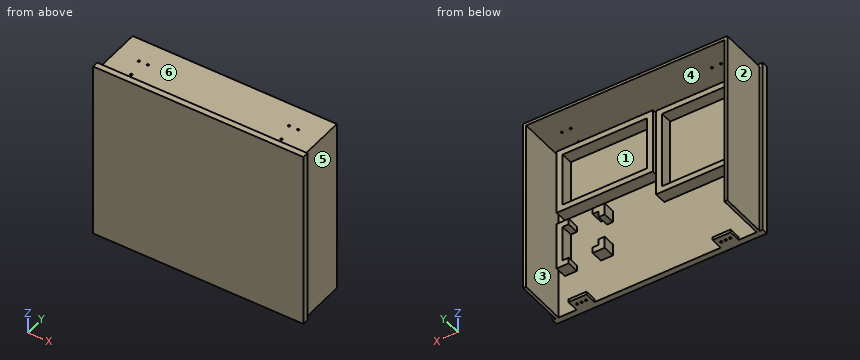
Autodesk Inventor part; units mm, degrees
ref_plane "YZ Plane" through (0, 0, 0) normal (1, 0, 0) x (0, 1, 0)
ref_plane "XZ Plane" through (0, 0, 0) normal (0, 1, 0) x (-1, 0, 0)
ref_plane "XY Plane" through (0, 0, 0) normal (0, 0, 1) x (1, 0, 0)
sketch "Sketch1" plane through (0, 0, 0) normal (0, 1, 0) x (-1, 0, 0)
  line L0 (-175, 150) -> (175, 150)
  line L1 (175, 150) -> (175, -150)
  line L2 (175, -150) -> (-175, -150)
  line L3 (-175, -150) -> (-175, 150)
  line L4 (-175, 150) -> (175, -150) construction
  line L5 (175, 150) -> (-175, -150) construction
  point P0 (0, 0)
  dimension "d0" = 350
  dimension "d1" = 300
extrude "Extrusion1" add sketch "Sketch1" along normal blind 10
sketch "Sketch2" plane through (0, 10, 0) normal (0, 1, 0) x (1, 0, 0)
  line L0 (175, 150) -> (-175, 150)
  line L1 (-175, 150) -> (-170, 150)
  line L2 (-170, 150) -> (-165, 150)
  line L3 (-165, 150) -> (-165, -145)
  line L4 (-165, -145) -> (-170, -145)
  line L5 (-170, -145) -> (-170, 150)
  line L6 (-170, -145) -> (170, -145)
  line L7 (170, -145) -> (170, -140)
  line L8 (170, -140) -> (-170, -140)
  line L9 (-170, -140) -> (-170, -145)
  line L10 (170, -140) -> (165, -140)
  line L11 (165, -140) -> (165, 150)
  line L12 (165, 150) -> (170, 150)
  line L13 (170, 150) -> (170, -140)
  point P0 (0, 0)
  point P1 (-170, 145)
  point P2 (170, 145)
  point P3 (-165, -140)
  point P4 (-165, -145)
  dimension "d5" = 5
  dimension "d6" = 5
  dimension "d7" = 5
extrude "Extrusion2" add sketch "Sketch2" along normal blind 80 contours L13 L8 L11 L0 | L7 L6 L3 L8 | L3 L8 L5 L0 | L3 L4 L5 L8
sketch "Sketch3" plane through (-175, 0, 150) normal (0, 0, 1) x (1, 0, 0)
  line L0 (5, 10) -> (5, 90)
  line L1 (5, 90) -> (50, 90)
  line L2 (340, 90) -> (10, 90)
  line L3 (50, 90) -> (50, 20)
  line L4 (345, 10) -> (345, 90)
  line L5 (345, 90) -> (300, 90)
  line L6 (300, 90) -> (300, 20)
  line L7 (350, 10) -> (345, 10)
  line L8 (350, 10) -> (350, 90)
  point P0 (175, 0)
  point P1 (307.5, 50)
  point P2 (292.5, 50)
  point P3 (42.5, 50)
  point P4 (57.5, 50)
  dimension "d10" = 45
  dimension "d11" = 70
  dimension "d12" = 45
  dimension "d13" = 70
sketch "Sketch4" plane through (0, 10, 0) normal (0, 1, 0) x (1, 0, 0)
  line L0 (165, 150) -> (-165, 150)
  line L1 (-165, 150) -> (-135, 150)
  line L2 (-135, 150) -> (-105, 150)
  line L3 (-105, 150) -> (-105, 145)
  line L4 (-105, 145) -> (-135, 145)
  line L5 (-135, 145) -> (-135, 150)
  line L6 (165, 150) -> (135, 150)
  line L7 (135, 150) -> (105, 150)
  line L8 (105, 150) -> (105, 145)
  line L9 (105, 145) -> (135, 145)
  line L10 (135, 145) -> (135, 150)
  point P0 (0, 0)
  dimension "d21" = 30
  dimension "d22" = 30
  dimension "d23" = 5
  dimension "d24" = 30
  dimension "d25" = 30
  dimension "d26" = 5
extrude "Extrusion3" add sketch "Sketch4" along normal blind 20
sketch "Sketch5" plane through (175, 0, -150) normal (0, 0, -1) x (-1, 0, 0)
  circle A0 centre (295, 20) radius 1.75
  line L0 (287.5, 20) -> (295, 20)
  point P0 (175, 0)
  point P1 (302.5, 20)
  point P2 (55, 20)
  point P3 (62.5, 20)
  point P4 (47.5, 20)
  dimension "d45" = 7.5
hole "Hole2" at (-120, 20, -150) at (-127.5, 20, -150) at (-112.5, 20, -150) at (120, 20, -150) at (112.5, 20, -150) at (127.5, 20, -150) direction (0, 0, 1) diameter 3.5 depth 10
hole "Hole3" at (-125, 20, 150) at (125, 20, 150) at (132.5, 50, 150) at (117.5, 50, 150) at (-132.5, 50, 150) at (-117.5, 50, 150) direction (0, 0, -1) diameter 3.5 depth 10
sketch "Sketch6" plane through (0, 10, 0) normal (0, 1, 0) x (1, 0, 0)
  line L0 (-165, -140) -> (165, -140)
  line L1 (165, -140) -> (215, -140) construction
  line L2 (-5.3553, -129.6447) -> (154.6447, -129.6447)
  line L3 (154.6447, -129.6447) -> (154.6447, -19.6447)
  line L4 (154.6447, -19.6447) -> (-5.3553, -19.6447)
  line L5 (-5.3553, -19.6447) -> (-5.3553, -129.6447)
  line L6 (-5.3553, -129.6447) -> (154.6447, -19.6447) construction
  line L7 (154.6447, -129.6447) -> (-5.3553, -19.6447) construction
  line L8 (4.6447, -119.6447) -> (144.6447, -119.6447)
  line L9 (144.6447, -119.6447) -> (144.6447, -29.6447)
  line L10 (144.6447, -29.6447) -> (4.6447, -29.6447)
  line L11 (4.6447, -29.6447) -> (4.6447, -119.6447)
  line L12 (4.6447, -119.6447) -> (144.6447, -29.6447) construction
  line L13 (144.6447, -119.6447) -> (4.6447, -29.6447) construction
  point P0 (0, 0)
  point P1 (74.6447, -74.6447)
  dimension "d51" = 160
  dimension "d52" = 110
  dimension "d70" = 140
  dimension "d71" = 90
sketch "Sketch7" plane through (0, 10, 0) normal (0, 1, 0) x (1, 0, 0)
  line L0 (-165, -140) -> (165, -140)
  line L1 (-165, -140) -> (-150.8579, -125.8579)
  line L2 (-165, -140) -> (-145, -140) construction
  line L3 (-150.8579, -125.8579) -> (-10.8579, -125.8579)
  line L4 (-10.8579, -125.8579) -> (-10.8579, 24.1421)
  line L5 (-10.8579, 24.1421) -> (-150.8579, 24.1421)
  line L6 (-150.8579, 24.1421) -> (-150.8579, -125.8579)
  line L7 (-150.8579, -50.8579) -> (-80.8579, -50.8579)
  line L8 (-140.8579, -115.8579) -> (-20.8579, -115.8579)
  line L9 (-20.8579, -115.8579) -> (-20.8579, 14.1421)
  line L10 (-20.8579, 14.1421) -> (-140.8579, 14.1421)
  line L11 (-140.8579, 14.1421) -> (-140.8579, -115.8579)
  line L12 (-140.8579, -115.8579) -> (-20.8579, 14.1421) construction
  line L13 (-20.8579, -115.8579) -> (-140.8579, 14.1421) construction
  line L14 (-140.8579, -115.8579) -> (-150.8579, -115.8579)
  line L15 (-5.3553, -19.6447) -> (154.6447, -19.6447)
  line L16 (154.6447, -19.6447) -> (154.6447, 0.3553)
  line L17 (154.6447, 0.3553) -> (74.6447, 0.3553)
  line L18 (74.6447, 0.3553) -> (74.6447, 80.3553)
  line L19 (74.6447, 80.3553) -> (154.6447, 80.3553)
  line L20 (154.6447, 80.3553) -> (154.6447, 0.3553)
  line L21 (84.6447, 70.3553) -> (144.6447, 70.3553)
  line L22 (144.6447, 70.3553) -> (144.6447, 10.3553)
  line L23 (144.6447, 10.3553) -> (84.6447, 10.3553)
  line L24 (84.6447, 10.3553) -> (84.6447, 70.3553)
  line L25 (84.6447, 70.3553) -> (144.6447, 10.3553) construction
  line L26 (144.6447, 70.3553) -> (84.6447, 10.3553) construction
  line L27 (94.645, 70.3553) -> (134.645, 70.3553)
  line L28 (134.645, 70.3553) -> (134.645, 80.3553)
  line L29 (94.645, 80.3553) -> (94.645, 70.3553)
  line L30 (94.645, 10.3553) -> (134.645, 10.3553)
  line L31 (134.645, 0.3553) -> (94.645, 0.3553)
  line L32 (94.645, 80.3553) -> (134.645, 80.3553)
  line L33 (94.645, 10.3553) -> (94.645, 0.3553)
  line L34 (134.645, 10.3553) -> (94.645, 10.3553)
  line L35 (134.645, 10.3553) -> (134.645, 0.3553)
  line L36 (94.645, 0.3553) -> (134.645, 0.3553)
  line L37 (84.6447, 60.355) -> (84.6447, 20.355)
  line L38 (84.6447, 20.355) -> (74.6447, 20.355)
  line L39 (74.6447, 60.355) -> (84.6447, 60.355)
  point P0 (0, 0)
  point P1 (-140.8579, -50.8579)
  point P2 (114.6447, 40.3553)
  dimension "d55" = 20
  dimension "d56" = 45
  dimension "d57" = 140
  dimension "d58" = 150
  dimension "d59" = 120
  dimension "d60" = 130
  dimension "d61" = 20
  dimension "d62" = 80
  dimension "d63" = 80
  dimension "d75" = 60
  dimension "d76" = 60
  dimension "d77" = 40
  dimension "d78" = 40
extrude "Extrusion6" add sketch "Sketch6" along normal blind 20
extrude "Extrusion7" add sketch "Sketch7" along normal blind 20 contours L6 L14 L8 L9 L10 L11 L7 L5 L4 L3 | L17 L35 L23 L22 L21 L28 L19 L20 | L17 L18 L38 L24 L23 L33 | L29 L21 L24 L39 L18 L19
properties part number "Venstre_bottom"
Input: part model. Units: mm. Frame: model coordinates. Face numbers are marked on the shaded views. A direction names the side the tool comes from. Coordinates: 2 decimals unless noted, no trailing zeros. Write each loop counter-clockwise with the first axis right and the second up, starting at its lowest first coordinate (ties: lowest second). Pieces come first, ordered by that corner, then holes. Notation, with made-up numbers: M 75.25,58.5 L 124.25,58.5 A31 ccw 124.25,94.5 Z; hole C 4,41 d3. An arc over 180 degrees is marked long. Answer as a JSON object with one key per item and string values. Group by question number.
(1) Mould query, pull axis Z, two halves, no side actions, for the marked faces 4, 5 and 6. Classes: pulls with the +Z half, pulls with the -Z half, needs draft (parallel to the pull), parting line crosses it, or undercut.
(2) Section C-C on x = 17. Output: boundary loops of the cut face in (y, z), plus the area to 3 significant figures.
(3) Section D-D on z = -85. Output: boundary loops of the cut face in (x, y), plus the area to 3 significant figures.
(4) Ray query, line 1 along X through (y, z) = (27, 59); line 2 along Z through (x, y) = (31.5, 23); line 3 along X through (y, z) = (50, 141). Return the intervals inside material, ascending. Write a range as [from, to].
(5) Contact query for flat-ended pins moving along their axis: P1, Ø5.5, axis at x = 127.5, y = 20, coming from the +Z side; P2, Ø4.5, axis at x = -132.5, y = 50, coming from the -Z side; P3, Ø1.5, axis at x = -127, z = -147.5, coming from the +Y side. Output: stop coordinate, or through.
(6) Section A-A on z = 93. Output: boundary loops of the cut face in (x, y).
(7) Set-up query: the marked faces 1, 2 and 3. Return all of +Z, -Z, +X, -X, +Y, -Y with unobstructed straight access to the full face (end or side cutting, diameter ignored); none if empty.
(8) Section B-B on y = 42. Output: boundary loops of the cut face in (x, z).
Result set:
{
 "1": {"face 4": "undercut", "face 5": "needs draft", "face 6": "pulls with the +Z half"},
 "2": {"outline": "M 0,-150 L 10,-150 L 10,19.64 L 30,19.64 L 30,29.64 L 10,29.64 L 10,119.64 L 30,119.64 L 30,129.64 L 10,129.64 L 10,140 L 90,140 L 90,145 L 10,145 L 10,150 L 0,150 Z", "area": "3,800 mm2"},
 "3": {"outline": "M -175,0 L 175,0 L 175,10 L 170,10 L 170,90 L 165,90 L 165,10 L -165,10 L -165,90 L -170,90 L -170,10 L -175,10 Z", "area": "4,300 mm2"},
 "4": {"line 1": "x = [-170, -165], [-20.86, -10.86], [-5.36, 4.64], [144.64, 154.64], [165, 170]", "line 2": "z = [19.64, 29.64], [119.64, 129.64], [140, 145]", "line 3": "x = [-170, -134.25], [-130.75, -119.25], [-115.75, 115.75], [119.25, 130.75], [134.25, 170]"},
 "5": {"P1": "stops at z = 145", "P2": "stops at z = 140", "P3": "stops at y = 30"},
 "6": {"outline": "M -175,0 L 175,0 L 175,10 L 170,10 L 170,90 L 165,90 L 165,10 L 154.64,10 L 154.64,30 L 144.64,30 L 144.64,10 L 4.64,10 L 4.64,30 L -5.36,30 L -5.36,10 L -10.86,10 L -10.86,30 L -20.86,30 L -20.86,10 L -165,10 L -165,90 L -170,90 L -170,10 L -175,10 Z"},
 "7": {"face 1": "+Y", "face 2": "+Z, -Z, -X, +Y", "face 3": "-Z, +Y"},
 "8": {"outline": "M -170,-150 L -165,-150 L -165,140 L 165,140 L 165,-150 L 170,-150 L 170,145 L -170,145 Z"}
}
